Autodesk Inventor part; units mm, degrees
ref_plane "YZ Plane" through (0, 0, 0) normal (1, 0, 0) x (0, 1, 0)
ref_plane "XZ Plane" through (0, 0, 0) normal (0, 1, 0) x (-1, 0, 0)
ref_plane "XY Plane" through (0, 0, 0) normal (0, 0, 1) x (1, 0, 0)
sketch "草图1" plane through (0, 0, 0) normal (0, 1, 0) x (-1, 0, 0)
  circle A0 centre (0, 0) radius 5
  circle A1 centre (0, 0) radius 2.5
  dimension "d0" = 10
  dimension "d1" = 5
extrude "拉伸1" add sketch "草图1" along normal blind 15
ref_plane "工作平面1" through (0, 7.5, 0) normal (0, 1, 0) x (1, 0, 0)
sketch "草图2" plane through (0, 7.5, 0) normal (0, 1, 0) x (1, 0, 0)
  line L0 (-5, 7) -> (5, 7)
  line L1 (5, 7) -> (5, 27)
  line L2 (5, 27) -> (-5, 27)
  line L3 (-5, 27) -> (-5, 7)
  circle A0 centre (0, 0) radius 5
  circle A1 centre (0, 0) radius 5
  line L4 (5, 0) -> (5, 7)
  circle A2 centre (0, 0) radius 5
  line L5 (-5, 0) -> (-5, 7)
  dimension "d4" = 10
  dimension "d5" = 20
  dimension "d6" = 7
  dimension "d7" = 10
  dimension "d8" = 5
extrude "拉伸2" add sketch "草图2" along normal mid plane 45 contours L3 L2 L1 L0 | L0 L4 A0 L5
sketch "草图3" plane through (-5, -15, -27) normal (-1, 0, 0) x (0, 0, 1)
  line L0 (27, 0) -> (0, 0)
  line L1 (0, 0) -> (0, 45)
  point P0 (27, 15)
  point P1 (10, 22.5)
  dimension "d11" = 22.5
  dimension "d12" = 10
hole "孔1" at (-5, 7.5, -17) direction (1, 0, 0) diameter 8.376 depth 27.3
properties part number "连接块2"
Can you work these out from the model? Positions are in its coordinate system, mm. A direction names the side the tool comes from. Round coordinates to 2 decimals unless told otherwise and drop trailing zeros. Write each loop counter-clockwise with the first axis right and the second up, starting at its lowest first coordinate (ties: lowest second). Pieces come first, ordered by that corner, then holes. Notation, with made-up numbers: M 53.25,-18 L 71.25,-18 A34 cw 71.25,17 Z; hole C 34,-29 d10. An arc over 180 degrees is marked long. Use a Markdown table: item, result.
Item 1: Which directions (+Z, -Z, +X, -X, +Y, -Y) give clear straight access to the entire face, cutting with the end or side of a thin tool? Please do faces 5 (the face through (0, -8, -5)), 6 (the face through (0.07, 9.1, -13.13)), 7 (the face through (0, 22, -5)).
Found:
| item | result |
|---|---|
| face 5 | +Z, -Y |
| face 6 | +X, -X |
| face 7 | +Z, +Y |
Item 2: For pin 1 Ø6.5 at (y, z) = (7.5, -17) entering from -X; pin 2 Ø3 at (x, z) = (-2, -0.5) entering from -Y; pin 3 Ø4 at (x, y) = (-3.5, 20.5) entering from +Z, each with a flat end and sliding along its axis, tell me the tip position at first contact or that it passes through.
Found:
| item | result |
|---|---|
| pin 1 | passes through |
| pin 2 | stops at y = 0 |
| pin 3 | stops at z = 0 |
Item 3: I want a section at C-C (z = 2). List the corners of the cut face in (x, y) for me.
Found:
| item | result |
|---|---|
| outline | M -4.58,0 L -1.5,0 L -1.5,15 L -4.58,15 Z; M 1.5,0 L 4.58,0 L 4.58,15 L 1.5,15 Z |
Item 4: I want a section at A-A (y = 7.5). List the corners of the cut face in (x, z) for me, and give its area (3 significant figures).
Found:
| item | result |
|---|---|
| outline | M -5,-27 L 5,-27 L 5,-21.19 L -5,-21.19 Z; M -5,-12.81 L 5,-12.81 L 5,0 A5 ccw -5,0 Z; hole C 0,0 d5 |
| area | 206 mm2 |
Item 5: I want a section at D-D (x = 2). List the corners of the cut face in (y, z) for me, and give its area (3 significant figures).
Found:
| item | result |
|---|---|
| outline | M -15,-27 L 30,-27 L 30,-4.58 L 15,-4.58 L 15,-1.5 L 0,-1.5 L 0,-4.58 L -15,-4.58 Z; M 0,1.5 L 15,1.5 L 15,4.58 L 0,4.58 Z; hole C 7.5,-17 d8.38 |
| area | 1,050 mm2 |
Item 6: We'd pull the mould along X, two halves only. Please class faces 1 (the face through (-2, 0, -2)), 2 (the face through (-5, 7, -11)), 3 (the face through (0, -15, -17)), 4 (the face through (0, 7, 5)): released by +X, released by -X, zero draft, split by the parting line, or undercut.
Found:
| item | result |
|---|---|
| face 1 | undercut |
| face 2 | released by -X |
| face 3 | zero draft |
| face 4 | split by the parting line |
Item 7: If I drill on line 1 along Y through (x, z) = (-1, -17); line 2 along Z through (x, y) = (-2.25, 7); line 3 along Z through (x, y) = (-2.75, 6.5), over which ranges is the centre line in solid material (lowest first)? Write a range as [from, to].
Found:
| item | result |
|---|---|
| line 1 | y = [-15, 3.31], [11.69, 30] |
| line 2 | z = [-27, -21.16], [-12.84, -1.09], [1.09, 4.47] |
| line 3 | z = [-27, -21.07], [-12.93, 4.18] |
Item 8: I want a section at B-B (x = 0). List the corners of the cut face in (y, z) for me, and give its area (3 significant figures).
Found:
| item | result |
|---|---|
| outline | M -15,-27 L 30,-27 L 30,-5 L 15,-5 L 15,-2.5 L 0,-2.5 L 0,-5 L -15,-5 Z; M 0,2.5 L 15,2.5 L 15,5 L 0,5 Z; hole C 7.5,-17 d8.38 |
| area | 1,010 mm2 |
